Geometry: see drawing. Coordinates: mm, zero at the bounding-box minimum. A direction names the side the tool comes from. Round coordinates to 2 decimals unless told otherwise and drop trailing zeros. Loops run counter-clockwise (first coordinate to the right, second up) from the corner with the lowest first, then second, coordinate; pieces in that order, holes last.
(1) Mould query, pull axis X, two halves, no side actions, for the marked faces 1, 2 and 3. Classes: pulls with the +X half, pulls with the -X half, needs draft (parallel to the pull), parting line crosses it, or undercut.
(2) Section D-D, the plane z = 1.5. Return the cut outline in (x, y), plus the area to 3 significant figures.
(3) Section A-A, the plane z = 17. Return the cut outline in (x, y).
(4) Section B-B, the plane x = 7. Return the cut outline in (y, z), plus the area to 3 significant figures.
(5) Section C-C, the plane y = 4.5. Return the cut outline in (x, z).
(6) Material intervals for probe 1 along Z at (x, y) = (7, 2.75); probe 2 along X at (y, z) = (3, 17); probe 3 along X at (y, z) = (4.5, 3), sorted ascending.
(7) Set-up query: the marked faces 4, 5 and 6. Return all of +Z, -Z, +X, -X, +Y, -Y with unobstructed straight access to the full face (end or side cutting, diameter ignored); none if empty.
(8) First-contact query: pin 1 Ø0.7 at (x, z) = (1.5, 9) entering from +Y; pin 2 Ø6 at (x, z) = (1.5, 6.5) entering from +Y; pin 3 Ø1.2 at (y, z) = (3, 14.5) entering from +X. Flat tips, straight axial feed; report the tip coordinate or a pass-through.
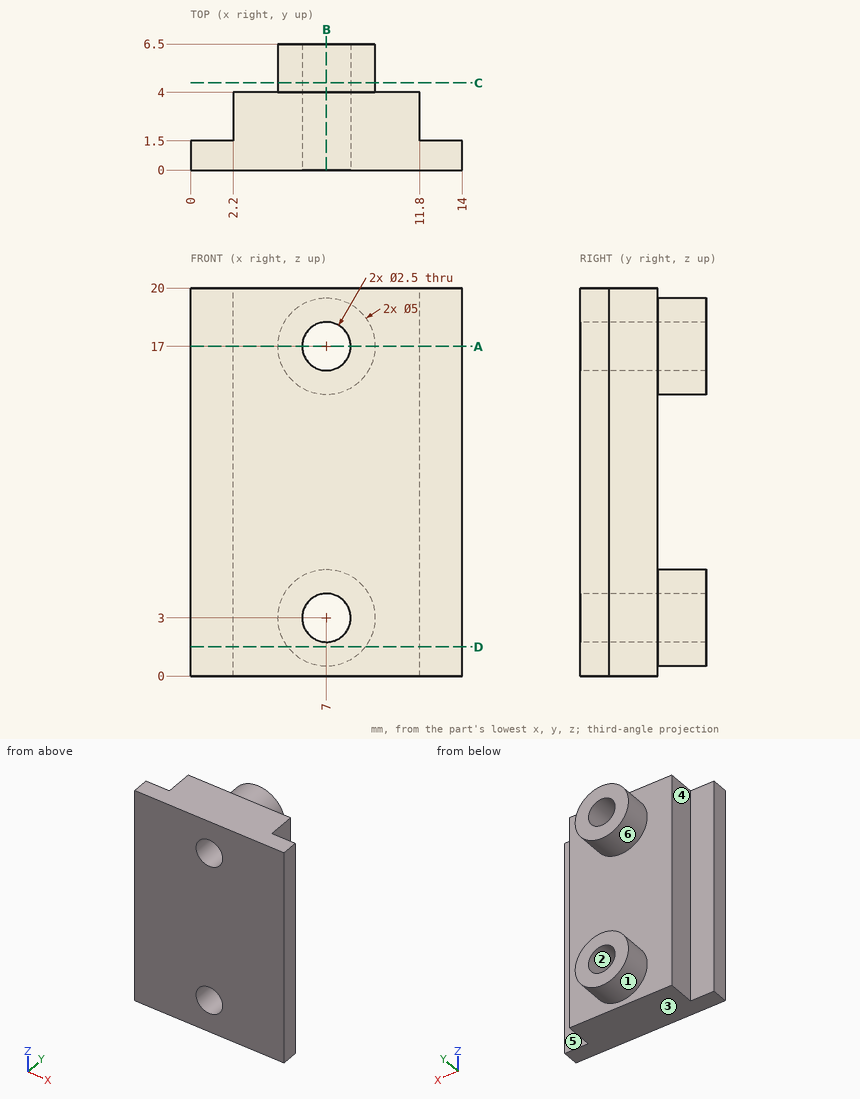
Output values:
1. face 1: parting line crosses it
1. face 2: undercut
1. face 3: needs draft
2. outline: (0, 0) - (14, 0) - (14, 1.5) - (11.8, 1.5) - (11.8, 4) - (9, 4) - (9, 6.5) - (5, 6.5) - (5, 4) - (2.2, 4) - (2.2, 1.5) - (0, 1.5) - close
2. area: 55.0 mm2
3. outline: (0, 0) - (5.75, 0) - (5.75, 6.5) - (4.5, 6.5) - (4.5, 4) - (2.2, 4) - (2.2, 1.5) - (0, 1.5) - close; (8.25, 0) - (14, 0) - (14, 1.5) - (11.8, 1.5) - (11.8, 4) - (9.5, 4) - (9.5, 6.5) - (8.25, 6.5) - close
4. outline: (0, 0) - (4, 0) - (4, 0.5) - (6.5, 0.5) - (6.5, 1.75) - (0, 1.75) - close; (0, 4.25) - (6.5, 4.25) - (6.5, 5.5) - (4, 5.5) - (4, 14.5) - (6.5, 14.5) - (6.5, 15.75) - (0, 15.75) - close; (0, 18.25) - (6.5, 18.25) - (6.5, 19.5) - (4, 19.5) - (4, 20) - (0, 20) - close
4. area: 72.5 mm2
5. outline: circle Ø5 at (7, 3); circle Ø5 at (7, 17); hole circle Ø2.5 at (7, 3); hole circle Ø2.5 at (7, 17)
6. probe 1: z = 0 to 1.75, 4.25 to 15.75, 18.25 to 20
6. probe 2: x = 2.2 to 5.75, 8.25 to 11.8
6. probe 3: x = 4.5 to 5.75, 8.25 to 9.5
7. face 4: +Z, -Z, -X, +Y
7. face 5: +Z, -Z, +X, +Y
7. face 6: +Y
8. pin 1: stops at y = 1.5
8. pin 2: stops at y = 4
8. pin 3: stops at x = 11.8
